Read the model definition and answer for the solid it produces. Units are mm, in the model's axes. A direction names the side the tool comes from. Coordinates: 2 decimals unless noted, no trailing zeros. Loops run counter-clockwise (first coordinate to the right, second up) from the corner with the lowest first, then second, coordinate; pieces in that order, holes last. Notation, with made-up numbers: M 67.25,-1 L 114.25,-1 A19 ccw 114.25,25 Z; hole C 72.25,2 d3. An arc over 180 degrees is marked long. Use one line per item in the form item = value. Start each with the question number.
1. The part is cut by section D-D (z = 51). Give the vertices of the cut face in (x, y), plus the area to 3 significant figures.
2. The part is cut by section B-B (x = -1). Give the vertices of the cut face in (y, z), plus the area to 3 significant figures.
3. Find the intervals of material crossed by probe 1 along Y at (x, z) = (10.5, 100.9); probe 2 along X at (y, z) = (-10.5, 102.75); probe 3 along Z at (x, y) = (-12.5, -1.5), in increasing order. Write a range as [from, to].
4. The part is cut by section A-A (z = 8.5). Give the vertices of the cut face in (x, y), plus the area to 3 significant figures.
5. A flat-ended cylindrical pin translates along its axis: pin 1 (1.2 mm diameter, centred on y = 11, z = 101, fed in from -X). Find the tip coordinate at first contact, or state that the pin passes through.
6. A tool of negligible diameter and unlimited length cuts with its end or side. For faces 4 (the flat face through (2.5, -11, 102)), 5 (the flat face through (-10, 8, 9)), 6 (the flat face through (-9, 0, 102)), 7 (the flat face through (-8, -11, 9)), from which of +Z, -Z, +X, -X, +Y, -Y can it reach the whole face along a straight path? Write none if from no direction.
7. The part is cut by section C-C (y = 4). Give the vertices of the cut face in (x, z).
8. For a pull along Z with two mould halves and no side action, classify faces 1 (the flat face through (-10, 0, 104)), 2 (the flat face through (-15, 0, 55)), 3 (the flat face through (-10, 7, 63)) as released by +Z, released by -Z, zero draft, split by the parting line, or undercut.
from build123d import *

# Parameters (mm, degrees)
F0_W      = 26
F0_H      = 26
F0_W_2    = 16
F0_H_2    = 16
F1_DEPTH  = 2
F2_DEPTH  = 100
F3_W      = 26
F3_H      = 26
F3_W_2    = 18
F3_H_2    = 18
F4_DEPTH  = 4
F5_W      = 5
F5_H      = 4
F6_DEPTH  = 4
F7_D      = 2.7
F7_DEPTH  = 4
F7_TIP    = 0.8111618357
F9_DEPTH  = 25
F10_W     = 3
F10_H     = 16
F11_DEPTH = 26
F12_W     = 4
F12_H     = 12
F13_DEPTH = 20
F14_W     = 16
F14_H     = 15
F15_DEPTH = 40
F16_W     = 16
F16_H     = 15
F17_DEPTH = 40


with BuildPart() as f1:
    # F0 (on Top) → F1 (new body)
    with BuildSketch(Plane.XY):
        Rectangle(F0_W, F0_H)
        Rectangle(F0_W_2, F0_H_2, mode=Mode.SUBTRACT)
        Rectangle(F0_W_2, F0_H_2)
    extrude(amount=F1_DEPTH)

    # F0 (on Top) → F2 (join)
    with BuildSketch(Plane.XY):
        Rectangle(F0_W, F0_H)
        Rectangle(F0_W_2, F0_H_2, mode=Mode.SUBTRACT)
    extrude(amount=F2_DEPTH)

    # F3 (on face) → F4 (join)
    with BuildSketch(Plane.XY.offset(100)):
        Rectangle(F3_W, F3_H)
        Rectangle(F3_W_2, F3_H_2, mode=Mode.SUBTRACT)
    extrude(amount=F4_DEPTH)

    # F5 (on face) → F6 (cut, through all)
    with BuildSketch(Plane.XY.offset(104)):
        with Locations((0, -11)):
            Rectangle(F5_W, F5_H)
        with Locations((0, 11)):
            Rectangle(F5_W, F5_H)
    extrude(amount=-F6_DEPTH, mode=Mode.SUBTRACT)

    # F7
    with Locations(Plane.XY.offset(104)):
        with Locations((-10.5, 10.5), (10.5, 10.5), (-10.5, -10.5), (10.5, -10.5)):
            Hole(F7_D / 2, depth=F7_DEPTH)
            with Locations((0, 0, -(F7_DEPTH + F7_TIP / 2))):  # 118° drill point
                Cone(0, F7_D / 2, F7_TIP, mode=Mode.SUBTRACT)

    # F0 (on Top) → F9 (cut)
    with BuildSketch(Plane.XY):
        Rectangle(F0_W_2, F0_H_2)
    extrude(amount=F9_DEPTH, mode=Mode.SUBTRACT)

    # F10 (on face) → F11 (join)
    with BuildSketch(Plane.XZ.offset(13)):
        with Locations((-14.5, 63)):
            Rectangle(F10_W, F10_H)
    extrude(amount=-F11_DEPTH)

    # F12 (on face) → F13 (cut)
    with BuildSketch(Plane.XZ.offset(13)):
        with Locations((-9, 63)):
            Rectangle(F12_W, F12_H)
    extrude(amount=-F13_DEPTH, mode=Mode.SUBTRACT)

    # F14 (on face) → F15 (cut)
    with BuildSketch(Plane.XZ.offset(13)):
        with Locations((0, 9.5)):
            Rectangle(F14_W, F14_H)
    extrude(amount=-F15_DEPTH, mode=Mode.SUBTRACT)

    # F16 (on face) → F17 (cut)
    with BuildSketch(Plane.YZ.offset(13)):
        with Locations((0, 9.5)):
            Rectangle(F16_W, F16_H)
    extrude(amount=-F17_DEPTH, mode=Mode.SUBTRACT)


solid = f1.part
Computed values:
q1.outline = M -13,-13 L 13,-13 L 13,13 L -13,13 Z; hole M -8,-8 L 8,-8 L 8,8 L -8,8 Z
q1.area = 420 mm²
q2.outline = M -13,0 L -8,0 L -8,2 L -13,2 Z; M -13,17 L -8,17 L -8,100 L -13,100 Z; M 8,0 L 13,0 L 13,2 L 8,2 Z; M 8,17 L 13,17 L 13,100 L 8,100 Z
q2.area = 850 mm²
q3.probe_1 = [-13, -11.85], [-9.15, 9.15], [11.85, 13]
q3.probe_2 = [-13, -11.85], [-9.15, -2.5], [2.5, 9.15], [11.85, 13]
q3.probe_3 = [0, 2], [17, 104]
q4.outline = M -13,-13 L -8,-13 L -8,-8 L -13,-8 Z; M -13,8 L -8,8 L -8,13 L -13,13 Z; M 8,-13 L 13,-13 L 13,-8 L 8,-8 Z; M 8,8 L 13,8 L 13,13 L 8,13 Z
q4.area = 100 mm²
q5.pin_1 = -13
q6.face_4 = +Z, +Y, -Y
q6.face_5 = +X, -X
q6.face_6 = +Z
q6.face_7 = +Y, -Y
q7.outline = M -16,55 L -13,55 L -13,17 L -8,17 L -8,57 L -11,57 L -11,69 L -8,69 L -8,100 L -9,100 L -9,104 L -13,104 L -13,71 L -16,71 Z; M -13,0 L -8,0 L -8,2 L -13,2 Z; M 8,0 L 13,0 L 13,2 L 8,2 Z; M 8,17 L 13,17 L 13,104 L 9,104 L 9,100 L 8,100 Z
q8.face_1 = released by +Z
q8.face_2 = released by -Z
q8.face_3 = undercut
